Answer from the drawing. Dimensions are ordinates in mm from the lowest x, y and z of the part. A direction names the side the tool comes from. Give positions to 0.01 mm unless a question says otherwise; leave off trailing zeros. Order: outer loops, then holes, each group sorted by start corner. A loop starts at its lowest first (then second) coordinate and runs counter-clockwise, first axis right, second up.
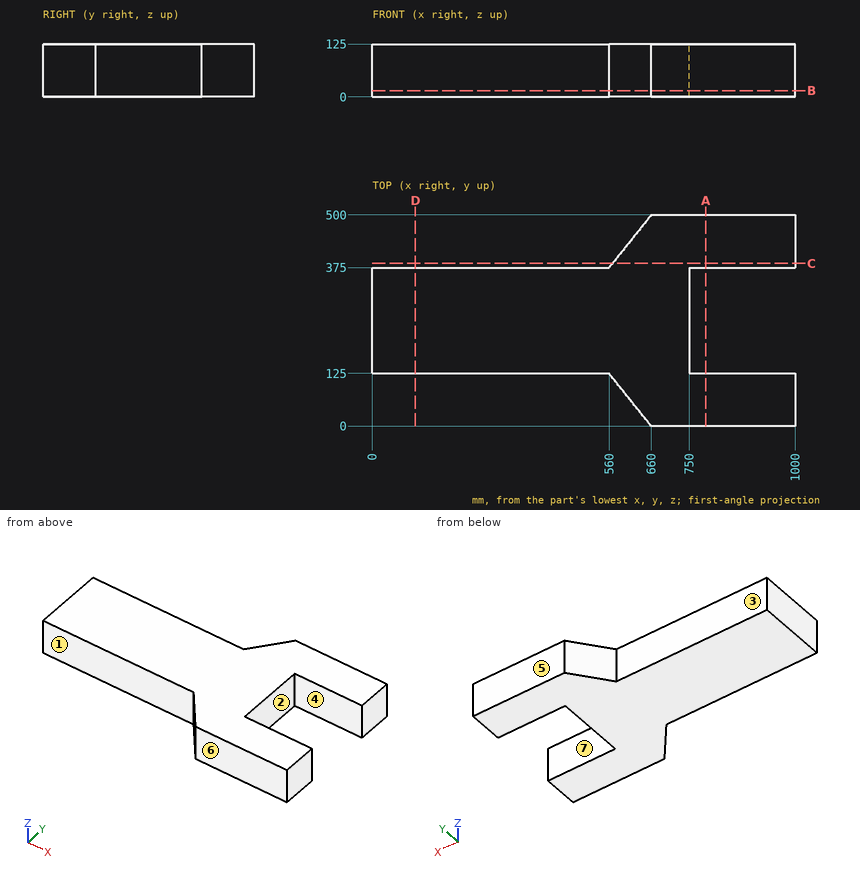
1) For a pull along Y with two mould halves and no side action, classify the marked faces 4, 5, 6 and 7 as released by +Y, released by -Y, zero draft, split by the parting line, or undercut.
Final values:
face 4: undercut
face 5: released by +Y
face 6: released by -Y
face 7: undercut
2) The part is cut by section B-B on z = 14.5. Determine the outline of the cut face in (x, y), and give its area (3 significant figures).
Final values:
outline: (0, 125) - (560, 125) - (660, 0) - (1000, 0) - (1000, 125) - (750, 125) - (750, 375) - (1000, 375) - (1000, 500) - (660, 500) - (560, 375) - (0, 375) - close
area: 285,000 mm2
3) The part is cut by section A-A on x = 789. Determine the outline of the cut face in (y, z).
Final values:
outline: (0, 0) - (125, 0) - (125, 125) - (0, 125) - close; (375, 0) - (500, 0) - (500, 125) - (375, 125) - close
4) The part is cut by section C-C on y = 385. Determine the outline of the cut face in (x, z).
Final values:
outline: (568, 0) - (1000, 0) - (1000, 125) - (568, 125) - close
5) Given pin 1 (6 mm diameter, centred on y = 93.5, z = 46, fed in from -X); pin 2 (1.5 mm diameter, centred on y = 306, z = 52, fed in from +X), each flat-ended and moving along its own axis, determine where each tip first touches the part or whether it passes through.
Final values:
pin 1: stops at x = 582.8
pin 2: stops at x = 750
6) The part is cut by section D-D on x = 102. Determine the outline of the cut face in (y, z).
Final values:
outline: (125, 0) - (375, 0) - (375, 125) - (125, 125) - close
7) A tool of negligible diameter and unlimited length cuts with its end or side. For the marked faces 1, 2 and 3, from which of +Z, -Z, +X, -X, +Y, -Y can it reach the whole face along a straight path? Write none if from no direction.
Final values:
face 1: +Z, -Z, -X, -Y
face 2: +Z, -Z, +X
face 3: +Z, -Z, -X, +Y
8) Consider L1, parallel to Y at x = 918, z = 60; L2, parallel to X at y = 137.5, z = 15; L3, parallel to Y at x = 198.5, z = 52. Determine where each line is inside the solid, lowest interval first.
Final values:
L1: y = 0 to 125, 375 to 500
L2: x = 0 to 750
L3: y = 125 to 375
